Verification items for this drawing (mm, ordinates from the low corner). Round coordinates to 2 decimals unless told otherwise and drop trailing zeros. Loops run counter-clockwise (first coordinate to the right, second up) from the corner with the lowest first, then second, coordinate; pieces in that order, holes last. Notation, with made-up numbers: (4, 29) -> (37, 29) arc R27 cw to (37, 59) -> close; hole circle Ø5 at (-21, -33). An arc over 180 degrees is marked (long way). One line per question, with ' | ' between items.
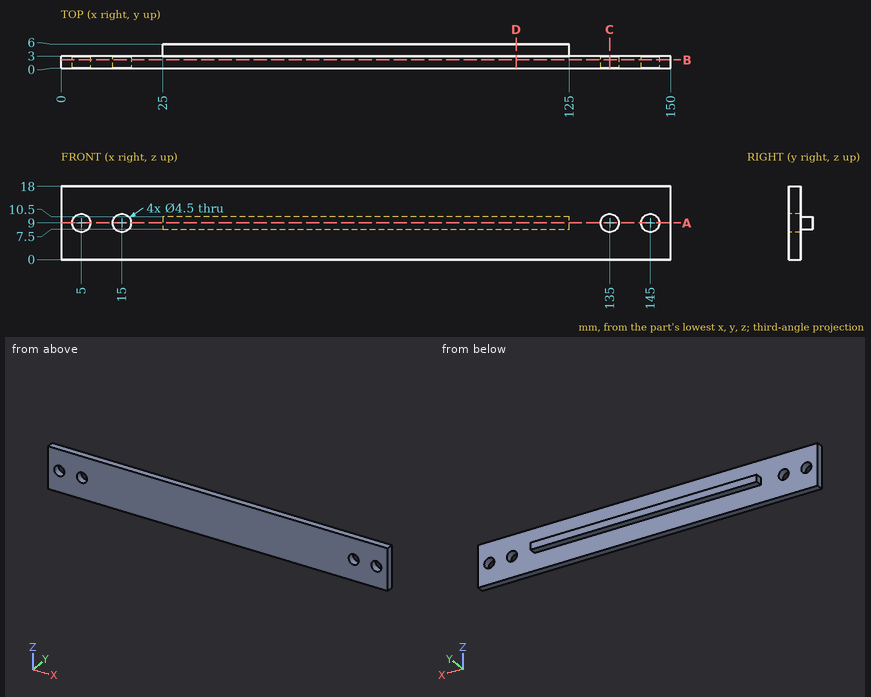
(1) Sectioned sample at D-D, the plane x = 112. Record the cut outline in (y, z).
Answer:
outline: (0, 0) -> (3, 0) -> (3, 7.5) -> (6, 7.5) -> (6, 10.5) -> (3, 10.5) -> (3, 18) -> (0, 18) -> close
(2) Sectioned sample at A-A, the plane z = 9. Record the cut outline in (x, y).
Answer:
outline: (0, 0) -> (2.75, 0) -> (2.75, 3) -> (0, 3) -> close; (7.25, 0) -> (12.75, 0) -> (12.75, 3) -> (7.25, 3) -> close; (17.25, 0) -> (132.75, 0) -> (132.75, 3) -> (125, 3) -> (125, 6) -> (25, 6) -> (25, 3) -> (17.25, 3) -> close; (137.25, 0) -> (142.75, 0) -> (142.75, 3) -> (137.25, 3) -> close; (147.25, 0) -> (150, 0) -> (150, 3) -> (147.25, 3) -> close
(3) Go/stop test with flat-tipped pins: pin 1 (2.5 mm diameter, centred on x = 56.5, y = 5, fed in from -Z); pin 2 (7 mm diameter, centred on x = 15, z = 9, fed in from +Y); pin 3 (3.5 mm diameter, centred on x = 135, z = 9, fed in from -Y); pin 4 (0.9 mm diameter, centred on y = 4.5, z = 9, fed in from -X). Record where each tip stops, or that it passes through.
Answer:
pin 1: stops at z = 7.5 | pin 2: stops at y = 3 | pin 3: passes through | pin 4: stops at x = 25
(4) Sectioned sample at B-B, the plane y = 2.1. Record the cut outline in (x, z).
Answer:
outline: (0, 0) -> (150, 0) -> (150, 18) -> (0, 18) -> close; hole circle Ø4.5 at (5, 9); hole circle Ø4.5 at (15, 9); hole circle Ø4.5 at (135, 9); hole circle Ø4.5 at (145, 9)
(5) Scan lines: probe 1 along Z at (x, y) = (145, 1.4); probe 2 along Y at (x, z) = (125, 10.75); probe 3 along Z at (x, y) = (42.5, 5.5). Record each from-to range of solid material in increasing order.
Answer:
probe 1: z = 0 to 6.75, 11.25 to 18 | probe 2: y = 0 to 3 | probe 3: z = 7.5 to 10.5
(6) Sectioned sample at C-C, the plane x = 135. Record the cut outline in (y, z), and give its area (3 significant figures).
Answer:
outline: (0, 0) -> (3, 0) -> (3, 6.75) -> (0, 6.75) -> close; (0, 11.25) -> (3, 11.25) -> (3, 18) -> (0, 18) -> close | area: 40.5 mm2
